Source: three-view drawing plus pictorial views. Frame: mm from the lowest corner of the part. Give positions to 0.01 mm unless a question says otherwise; leave off trailing zeros. Loops run counter-clockwise (first coordinate to the right, second up) from the corner with the lowest first, then second, coordinate; pieces in that order, holes last. Notation, with made-up numbers: M -25.75,32 L 9.25,32 A35 cw 9.25,67 Z; hole C 83,48.5 d4. An arc over 180 degrees is marked long. Put each result on its own line as item: value. Start each with the question number.
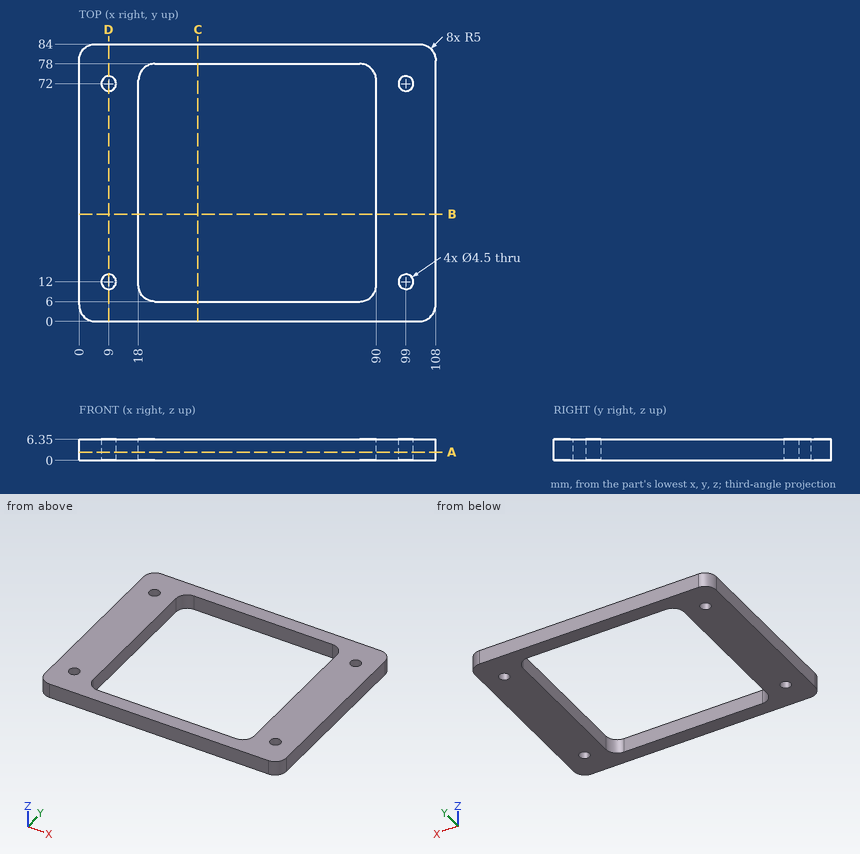
1. Section B-B, the plane y = 32.5. Output: boundary loops of the cut face in (x, z).
2. Contact query for a flat-ended pin moving along its axis: pin 1 (10 mm diameter, centred on x = 71, y = 13, fed in from -Z). Output: stop coordinate, or through.
3. Ray query, line 1 (Y direction, x = 9, z = 3); line 2 (X direction, y = 72, z = 2.5); line 3 (Y direction, x = 51, z = 4.5). Return the intervals inside material, ascending.
4. Section A-A, the plane z = 2.5. Output: boundary loops of the cut face in (x, y), plus the area to 3 significant figures.
5. Section C-C, the plane x = 36. Output: boundary loops of the cut face in (y, z).
6. Section D-D, the plane x = 9. Output: boundary loops of the cut face in (y, z).
Results found:
1. outline: M 0,0 L 18,0 L 18,6.35 L 0,6.35 Z; M 90,0 L 108,0 L 108,6.35 L 90,6.35 Z
2. pin 1: through
3. line 1: 0 to 9.75, 14.25 to 69.75, 74.25 to 84
3. line 2: 0 to 6.75, 11.25 to 18, 90 to 96.75, 101.25 to 108
3. line 3: 0 to 6, 78 to 84
4. outline: M 0,5 A5 ccw 5,0 L 103,0 A5 ccw 108,5 L 108,79 A5 ccw 103,84 L 5,84 A5 ccw 0,79 Z; hole C 9,12 d4.5; hole C 9,72 d4.5; hole M 18,11 A5 ccw 23,6 L 85,6 A5 ccw 90,11 L 90,73 A5 ccw 85,78 L 23,78 A5 ccw 18,73 Z; hole C 99,12 d4.5; hole C 99,72 d4.5
4. area: 3,820 mm²
5. outline: M 0,0 L 6,0 L 6,6.35 L 0,6.35 Z; M 78,0 L 84,0 L 84,6.35 L 78,6.35 Z
6. outline: M 0,0 L 9.75,0 L 9.75,6.35 L 0,6.35 Z; M 14.25,0 L 69.75,0 L 69.75,6.35 L 14.25,6.35 Z; M 74.25,0 L 84,0 L 84,6.35 L 74.25,6.35 Z
